Verification items for the finished model (mm, model axes). Face numbers are marked on the shaded views. A direction names the side the tool comes from. Coordinates: 2 decimals unless noted, no trailing zeros. Loops run counter-clockwise (first coordinate to the right, second up) from the corner with the lowest first, then second, coordinate; pieces in that order, holes last. Notation, with made-up numbers: (30.25, 9.25) -> (41.25, 9.25) arc R23 ccw to (41.25, 23.25) -> close; hole circle Ø5 at (62, 31). An arc over 180 degrees is marked (long way). Answer as a JSON object with one key per item and string values. Group by question number.
Q1. Gauge pin test, flat ends, axial feed: pin 1 Ø1.5 at (y, z) = (-43, 2.5) entering from +X; pin 2 Ø2.5 at (x, y) = (-4.5, -25.77) entering from +Z; pin 3 Ø1.5 at (x, z) = (-0.5, 0.5) entering from -Y. Record the tip position at first contact, or that the pin passes through.
Q2. Cross-section at D-D on x = 8.25. Record the boundary of the cut face in (y, z).
Q3. Scan lines: L1, parallel to Y at x = 0, z = 0.7 (3 decimals); L2, parallel to X at y = -27, z = 1.95; L3, parallel to Y at x = -2.75, z = 2.6. Record each from-to range of solid material in increasing order.
Q4. Cross-section at A-A on x = 0. Record the boundary of the cut face in (y, z) (3 decimals), and give its area (4 significant figures).
Q5. Cross-section at C-C on z = 2.4. Record the boundary of the cut face in (x, y) (3 decimals).
Q6. Cross-section at B-B on y = -54. Record the boundary of the cut face in (x, z).
Q7. Release check for a two-part mould opening along Y. For the marked faces 3, 4, 5 and 6 record: released by +Y, released by -Y, zero draft, split by the parting line, or undercut.
Q8. Set-up check for the marked faces 1 and 2: record each of +Z, -Z, +X, -X, +Y, -Y from which the full face is reachable in a straight line by a thin tool's end or side.
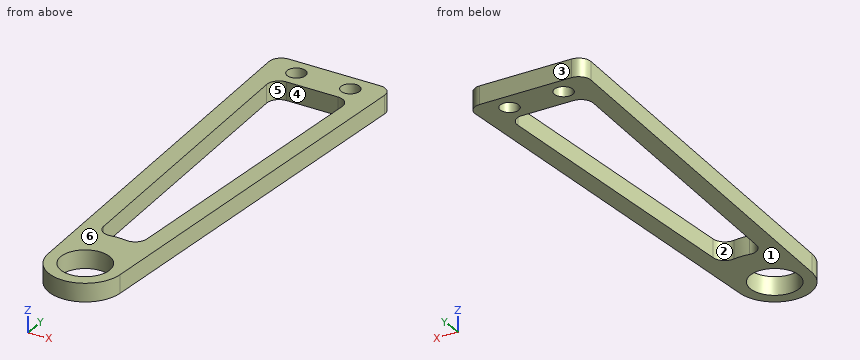
```python
from build123d import *

# Parameters (mm, degrees)
SKETCH_1_R          = 11
SKETCH_1_R_2        = 3.5
SKETCH_1_R_3        = 1.01
SKETCH_1_R_4        = 6
SKETCH_1_R_5        = 4.025
EXTRUDE_1_DEPTH     = 3
SKETCH_2_R          = 1.525
EXTRUDE_2_DEPTH     = 3
SKETCH_3_W          = 24.553172336
SKETCH_3_H          = 36.576889883
CUT_EXTRUDE_1_DEPTH = 10
FILLET_1_R          = 2


with BuildPart() as part:
    # 草图1 → 凸台-拉伸1 (new body)
    # profile 1 of 3: a face of its own
    with BuildSketch(Plane.XY):
        with BuildLine():
            ThreePointArc((10.983011573, -0.611111111), (0, -11), (-10.983011573, -0.611111111))
            Line((-10.983011573, -0.611111111), (-5.990733585, -90.333333333))
            ThreePointArc((-5.990733585, -90.333333333), (-0.166731054, -84.002317051), (6, -90))
            ThreePointArc((6, -90), (5.997682949, -90.166731054), (5.990733585, -90.333333333))
            Line((5.990733585, -90.333333333), (10.983011573, -0.611111111))
        make_face()
        with BuildLine():
            Line((-3.466771313, -81.694489982), (-7.418369738, -10.675569794))
            ThreePointArc((-7.418369738, -10.675569794), (0, -13), (7.418369738, -10.675569794))
            Line((7.418369738, -10.675569794), (3.466771313, -81.694489982))
            ThreePointArc((3.466771313, -81.694489982), (0, -81), (-3.466771313, -81.694489982))
        make_face(mode=Mode.SUBTRACT)
    # profile 2 of 3: a face of its own
    with BuildSketch(Plane.XY):
        Circle(SKETCH_1_R)
        Circle(SKETCH_1_R_2, mode=Mode.SUBTRACT)
        with Locations((-2.75, 4.763139721)):
            Circle(SKETCH_1_R_3, mode=Mode.SUBTRACT)
        with Locations((-2.75, -4.763139721)):
            Circle(SKETCH_1_R_3, mode=Mode.SUBTRACT)
        with Locations((5.5, 0)):
            Circle(SKETCH_1_R_3, mode=Mode.SUBTRACT)
    # profile 3 of 3: a face of its own
    with BuildSketch(Plane.XY):
        with Locations((0, -90)):
            Circle(SKETCH_1_R_4)
        with Locations((0, -90)):
            Circle(SKETCH_1_R_5, mode=Mode.SUBTRACT)
    extrude(amount=EXTRUDE_1_DEPTH)

    # 草图2 → 凸台-拉伸2 (add)
    with BuildSketch(Plane.XY.offset(3)):
        Polygon((-6.745155967, -22.774702841), (6.745155967, -22.774702841), (6.411307036, -28.774702841), (-6.411307036, -28.774702841), align=None)
        with Locations((-4.5, -25.774702841)):
            Circle(SKETCH_2_R, mode=Mode.SUBTRACT)
        with Locations((4.5, -25.774702841)):
            Circle(SKETCH_2_R, mode=Mode.SUBTRACT)
    extrude(amount=-EXTRUDE_2_DEPTH)

    # 草图3 → 切除-拉伸1 (cut)
    with BuildSketch(Plane.XY.offset(3)):
        with Locations((0.16395552, -4.486257899)):
            Rectangle(SKETCH_3_W, SKETCH_3_H)
    extrude(amount=-CUT_EXTRUDE_1_DEPTH, mode=Mode.SUBTRACT)

    # 圆角1
    fillet_1_edges = [part.edges().sort_by_distance(p)[0] for p in [
        (-3.466771313, -81.694489982, 1.5),
        (3.466771313, -81.694489982, 1.5),
        (6.411307036, -28.774702841, 1.5),
        (-6.411307036, -28.774702841, 1.5),
        (-9.749796341, -22.774702841, 1.5),
        (9.749796341, -22.774702841, 1.5),
    ]]
    fillet(fillet_1_edges, radius=FILLET_1_R)


solid = part.part
```
Computed values:
{
 "1": {"pin 1": "stops at x = 8.67", "pin 2": "passes through", "pin 3": "stops at y = -96"},
 "2": {"outline": "(-49.73, 0) -> (-22.87, 0) -> (-22.87, 3) -> (-49.73, 3) -> close"},
 "3": {"L1": "y = -96 to -94.025, -85.975 to -81, -28.775 to -22.775", "L2": "x = -9.51 to -5.41, -3.59 to 3.59, 5.41 to 9.51", "L3": "y = -95.33 to -92.94, -87.06 to -80.76, -28.77 to -22.77"},
 "4": {"outline": "(-96, 0) -> (-94.025, 0) -> (-94.025, 3) -> (-96, 3) -> close; (-85.975, 0) -> (-81, 0) -> (-81, 3) -> (-85.975, 3) -> close; (-28.775, 0) -> (-22.775, 0) -> (-22.775, 3) -> (-28.775, 3) -> close", "area": "38.85 mm²"},
 "5": {"outline": "(-9.632, -24.886) -> (-5.991, -90.333) arc R6 ccw to (5.991, -90.333) -> (9.632, -24.886) arc R2 ccw to (7.635, -22.775) -> (-7.635, -22.775) arc R2 ccw to start; hole (-6.294, -30.886) -> (-3.604, -79.229) arc R2 ccw to (-1.315, -81.097) arc R9 cw to (1.315, -81.097) arc R2 ccw to (3.604, -79.229) -> (6.294, -30.886) arc R2 ccw to (4.297, -28.775) -> (-4.297, -28.775) arc R2 ccw to start; hole circle Ø3.05 at (-4.5, -25.775); hole circle Ø8.05 at (0, -90); hole circle Ø3.05 at (4.5, -25.775)"},
 "6": {"outline": "(-8.01, 0) -> (-5.01, 0) -> (-5.01, 3) -> (-8.01, 3) -> close; (5.01, 0) -> (8.01, 0) -> (8.01, 3) -> (5.01, 3) -> close"},
 "7": {"face 3": "released by +Y", "face 4": "undercut", "face 5": "undercut", "face 6": "zero draft"},
 "8": {"face 1": "-Z, +X, -X, +Y, -Y", "face 2": "+Z, -Z"}
}
